```python
from build123d import *

# Parameters (mm, degrees)
F1_DEPTH = 11.4
F3_DEPTH = 5.4
F5_DEPTH = 7.4


with BuildPart() as f1:
    # F0 (on Front) → F1 (new body)
    with BuildSketch(Plane.XZ):
        with BuildLine():
            ThreePointArc((0, 10), (2.9289321881, 2.9289321881), (10, 0))
            Line((10, 0), (65, 0))
            ThreePointArc((65, 0), (72.0710678119, 2.9289321881), (75, 10))
            Line((75, 10), (75, 65))
            ThreePointArc((75, 65), (72.0710678119, 72.0710678119), (65, 75))
            Line((65, 75), (10, 75))
            ThreePointArc((10, 75), (2.9289321881, 72.0710678119), (0, 65))
            Line((0, 65), (0, 10))
        make_face()
        with BuildLine():
            ThreePointArc((1.7, 65), (4.1310137162, 70.8689862838), (10, 73.3))
            Line((10, 73.3), (65, 73.3))
            ThreePointArc((65, 73.3), (70.8689862838, 70.8689862838), (73.3, 65))
            Line((73.3, 65), (73.3, 10))
            ThreePointArc((73.3, 10), (70.8689862838, 4.1310137162), (65, 1.7))
            Line((65, 1.7), (10, 1.7))
            ThreePointArc((10, 1.7), (4.1310137162, 4.1310137162), (1.7, 10))
            Line((1.7, 10), (1.7, 65))
        make_face(mode=Mode.SUBTRACT)
    extrude(amount=F1_DEPTH)

    # F2 (on face) → F3 (join)
    with BuildSketch(Plane.XZ.offset(11.4)):
        with BuildLine():
            ThreePointArc((10, 73.3), (4.1310137162, 70.8689862838), (1.7, 65))
            Line((1.7, 65), (1.7, 10))
            ThreePointArc((1.7, 10), (4.1310137162, 4.1310137162), (10, 1.7))
            Line((10, 1.7), (65, 1.7))
            ThreePointArc((65, 1.7), (70.8689862838, 4.1310137162), (73.3, 10))
            Line((73.3, 10), (73.3, 65))
            ThreePointArc((73.3, 65), (70.8689862838, 70.8689862838), (65, 73.3))
            Line((65, 73.3), (10, 73.3))
        make_face()
    extrude(amount=-F3_DEPTH)

    # F4 (on face) → F5 (join)
    with BuildSketch(Plane.XZ.offset(11.4)):
        with BuildLine():
            Line((64, 69), (11, 69))
            ThreePointArc((11, 69), (7.4644660941, 67.5355339059), (6, 64))
            Line((6, 64), (6, 11))
            ThreePointArc((6, 11), (7.4644660941, 7.4644660941), (11, 6))
            Line((11, 6), (64, 6))
            ThreePointArc((64, 6), (67.5355339059, 7.4644660941), (69, 11))
            Line((69, 11), (69, 64))
            ThreePointArc((69, 64), (67.5355339059, 67.5355339059), (64, 69))
        make_face()
    extrude(amount=F5_DEPTH)


solid = f1.part
```
Input: part model. Units: mm. Frame: model coordinates. A direction names the side the tool comes from. Give positions to 0.01 mm unless a question says otherwise; leave off trailing zeros. Order: outer loops, then holes, each group sorted by start corner. A loop starts at its lowest first (then second) coordinate and runs counter-clockwise, first axis right, second up. Notation, with made-up numbers: (-34, 33) - (5, 33) arc R12 ccw to (5, 44) - close; hole circle Ø7 at (-22.5, -26.75). An arc over 180 degrees is marked (long way). Put each result on its own line as item: value.
Item 1: Ray query, L1, parallel to X at y = -1.75, z = 15; L2, parallel to Y at x = 70, z = 67.5. Return the intervals inside material, ascending. Write a range as from..to.
Found:
L1: x = 0..1.7, 73.3..75
L2: y = -11.4..-6
Item 2: Section query A-A, the plane y = -9.5. Return loops of the section in (x, z).
Found:
outline: (0, 10) arc R10 ccw to (10, 0) - (65, 0) arc R10 ccw to (75, 10) - (75, 65) arc R10 ccw to (65, 75) - (10, 75) arc R10 ccw to (0, 65) - close
Item 3: Draft query along X for faces 1 (the flat face through (37, -15, 6)), 2 (the flat face through (37, -6, 38)), 3 (the cylindrical face through (68, -15, 67)). Return one class per face: +X half, -X half, draft (parallel to the pull), parting line (faces both ways), or undercut.
Found:
face 1: draft
face 2: undercut
face 3: +X half
Item 4: Access query for faces 4 (the flat face through (69, -15, 37)), 5 (the cylindrical face through (4.196, -2.958, 4.067)), 6 (the cylindrical face through (67, -15, 7)), 7 (the flat face through (70, -11.4, 38)). Directions: +Z, -Z, +X, -X, +Y, -Y. A direction counts if a zero-diameter tool reaches every point of the face in a straight line with its end or side. Return the directions, or none.
Found:
face 4: +Z, -Z, +X, -Y
face 5: +Y
face 6: -Z, +X, -Y
face 7: -Y
Item 5: Contact query for flat-ended pins moving along their axis: pin 1 (6 mm diameter, centred on y = -14.5, z = 39.5, fed in from +X); pin 2 (3.5 mm diameter, centred on y = -14, z = 36.5, fed in from -X); pin 3 (4 mm diameter, centred on x = 43, z = 17, fed in from +Y); pin 4 (5 mm diameter, centred on y = -3.5, z = 35.5, fed in from -X). Output: stop coordinate, or through.
Found:
pin 1: stops at x = 69
pin 2: stops at x = 6
pin 3: stops at y = -6
pin 4: stops at x = 0
Item 6: Section query C-C, the plane z = 16.5. Return loops of the section in (x, y).
Found:
outline: (0, -11.4) - (6, -11.4) - (6, -18.8) - (69, -18.8) - (69, -11.4) - (75, -11.4) - (75, 0) - (73.3, 0) - (73.3, -6) - (1.7, -6) - (1.7, 0) - (0, 0) - close
Item 7: Section query D-D, the plane x = 12.5. Return loops of the section in (y, z).
Found:
outline: (-18.8, 6) - (-11.4, 6) - (-11.4, 0) - (0, 0) - (0, 1.7) - (-6, 1.7) - (-6, 73.3) - (0, 73.3) - (0, 75) - (-11.4, 75) - (-11.4, 69) - (-18.8, 69) - close
Item 8: Section query B-B, the plane y = -2. Return loops of the section in (x, z), then the cut area to 3 significant figures.
Found:
outline: (0, 10) arc R10 ccw to (10, 0) - (65, 0) arc R10 ccw to (75, 10) - (75, 65) arc R10 ccw to (65, 75) - (10, 75) arc R10 ccw to (0, 65) - close; hole (1.7, 10) arc R8.3 ccw to (10, 1.7) - (65, 1.7) arc R8.3 ccw to (73.3, 10) - (73.3, 65) arc R8.3 ccw to (65, 73.3) - (10, 73.3) arc R8.3 ccw to (1.7, 65) - close
area: 472 mm^2
